from build123d import *

# Parameters (mm, degrees)
SKETCH4_W          = 10.2
SKETCH4_H          = 12.5
CUT_EXTRUDE1_DEPTH = 6.6
SKETCH6_R          = 4.3
CUT_EXTRUDE2_DEPTH = 19.869552194
CHAMFER2_SIZE      = 0.5


with BuildPart() as part:
    # Sketch4 → Revolve1 (revolve)
    with BuildSketch(Plane(origin=(0, 0, 0), x_dir=(0, 0, -1), z_dir=(1, 0, 0)), mode=Mode.PRIVATE) as revolve1_sk:
        with Locations((-5.1, 6.25)):
            Rectangle(SKETCH4_W, SKETCH4_H)
    revolve(revolve1_sk.sketch.rotate(Axis((0, 0, 10.2), (0, 0, -1)), 180), axis=Axis((0, 0, 10.2), (0, 0, -1)))

    # Sketch5 → Cut-Extrude1 (cut)
    with BuildSketch(Plane.XY.offset(10.2)):
        Polygon((0, -7.67875858), (6.65, -3.83937929), (6.65, 3.83937929), (0, 7.67875858), (-6.65, 3.83937929), (-6.65, -3.83937929), align=None)
    extrude(amount=-CUT_EXTRUDE1_DEPTH, mode=Mode.SUBTRACT)

    # Sketch6 → Cut-Extrude2 (cut, through all)
    with BuildSketch(Plane.XY.offset(3.6)):
        Circle(SKETCH6_R)
    extrude(amount=-CUT_EXTRUDE2_DEPTH, mode=Mode.SUBTRACT)

    # Chamfer2
    chamfer2_edges = [part.edges().sort_by_distance(p)[0] for p in [
        (-3.325, -5.759068935, 10.2),
        (3.325, -5.759068935, 10.2),
        (6.65, 0, 10.2),
        (3.325, 5.759068935, 10.2),
        (-3.325, 5.759068935, 10.2),
        (-6.65, 0, 10.2),
        (-4.3, 0, 0),
        (0, 12.5, 0),
        (0, 12.5, 10.2),
    ]]
    chamfer(chamfer2_edges, length=CHAMFER2_SIZE)


solid = part.part
Work out the finished part from the listing and answer in its coordinate system (mm). A direction names the side the tool comes from. Give positions to 0.01 mm unless a question says otherwise; leave off trailing zeros. Order: outer loops, then holes, each group sorted by start corner. A loop starts at its lowest first (then second) coordinate and runs counter-clockwise, first axis right, second up. Notation, with made-up numbers: (18.5, 26.25) - (31.5, 26.25) arc R21 cw to (31.5, 56.25) - close; hole circle Ø3 at (7, 31.5). An arc over 180 degrees is marked (long way). Answer as CSV lines item,"result". Start each with the question number.
Q1. The part is cut by section C-C (z = 2). Write down the section's boundary in (x, y).
Q2. The mould has two halves that part along Y. Classify faces 1 (the face through (-3.755, -11.923, 5.036)), 2 (the face through (5, -6, 10.2)), 3 (the face through (3.498, 5.944, 9.946)): +Y half, -Y half, draft (parallel to the pull), parting line (faces both ways), or undercut.
Q3. Find the intervals of material crossed by L1, parallel to X at y = -4, z = 4.5; L2, parallel to X at y = 1.75, z = 4.5; L3, parallel to Y at x = 0.5, z = 8.5, in increasing order. Write a range as [from, to].
Q4. The part is cut by section B-B (y = 0). Write down the section's boundary in (x, z), then the cut area to 3 significant figures.
Q5. The part is cut by section A-A (z = 7). Write down the section's boundary in (x, y), then the cut area to 3 significant figures.
Q6. For faces 4 (the face through (-4.296, 0.189, 2.072)), 5 (the face through (3.278, -5.786, 6.693)), determine the directions among +Z, -Z, +X, -X, +Y, -Y from which every point of the face is accessible in a straight line to the end or side of a thin tool.
Q7. Given pin 1 Ø5 at (y, z) = (8, 3) entering from -X (3 decimals); pin 2 Ø1.5 at (x, z) = (-1, 1) entering from -Y; pin 3 Ø10 at (x, y) = (0, 0) entering from +Z, each flat-ended and moving along its own axis, determine where each tip first touches the part or whether it passes through.
Check result:
1,outline,"circle Ø25 at (0, 0); hole circle Ø8.6 at (0, 0)"
2,face 1,"parting line"
2,face 2,"draft"
2,face 3,"undercut"
3,L1,"x = [-11.84, -6.37], [6.37, 11.84]"
3,L2,"x = [-12.38, -6.65], [6.65, 12.38]"
3,L3,"y = [-12.49, -7.39], [7.39, 12.49]"
4,outline,"(-12.5, 0.5) - (-12, 0) - (-4.8, 0) - (-4.3, 0.5) - (-4.3, 3.6) - (-6.65, 3.6) - (-6.65, 9.7) - (-7.15, 10.2) - (-12, 10.2) - (-12.5, 9.7) - close; (4.3, 0.5) - (4.8, 0) - (12, 0) - (12.5, 0.5) - (12.5, 9.7) - (12, 10.2) - (7.15, 10.2) - (6.65, 9.7) - (6.65, 3.6) - (4.3, 3.6) - close"
4,area,"135 mm²"
5,outline,"circle Ø25 at (0, 0); hole (-6.65, -3.84) - (0, -7.68) - (6.65, -3.84) - (6.65, 3.84) - (0, 7.68) - (-6.65, 3.84) - close"
5,area,"338 mm²"
6,face 4,"+Z, -Z"
6,face 5,"+Z"
7,pin 1,"stops at x = -11.225"
7,pin 2,"stops at y = -12.5"
7,pin 3,"stops at z = 3.6"
